Can you work these out from the model? Positions are in its coordinate system, mm. Round coordinates to 2 decimals unless told otherwise and drop trailing zeros. Loops run counter-clockwise (first coordinate to the right, second up) from the corner with the lowest first, then second, coordinate; pieces in that order, holes last.
from build123d import *

# Parameters (mm, degrees)
F0_R     = 1.2446
F0_R_2   = 1.2192
F0_R_3   = 4.445
F1_DEPTH = 1.016


with BuildPart() as f1:
    # F0 (on Top) → F1 (new body)
    with BuildSketch(Plane.XY):
        with BuildLine():
            ThreePointArc((13.305479, -78.509091), (15.141437, -76.814431), (17.563232, -76.2))
            Line((17.563232, -76.2), (17.145, -76.2))
            ThreePointArc((17.145, -76.2), (20.737102, -74.712102), (22.225, -71.12))
            Line((22.225, -71.12), (22.225, 71.12))
            ThreePointArc((22.225, 71.12), (20.737102, 74.712102), (17.145, 76.2))
            Line((17.145, 76.2), (17.563232, 76.2))
            ThreePointArc((17.563232, 76.2), (15.141437, 76.814431), (13.305479, 78.509091))
            ThreePointArc((13.305479, 78.509091), (0, 85.725), (-13.305479, 78.509091))
            ThreePointArc((-13.305479, 78.509091), (-15.141437, 76.814431), (-17.563232, 76.2))
            Line((-17.563232, 76.2), (-17.145, 76.2))
            ThreePointArc((-17.145, 76.2), (-20.737102, 74.712102), (-22.225, 71.12))
            Line((-22.225, 71.12), (-22.225, -71.12))
            ThreePointArc((-22.225, -71.12), (-20.737102, -74.712102), (-17.145, -76.2))
            Line((-17.145, -76.2), (-17.563232, -76.2))
            ThreePointArc((-17.563232, -76.2), (-15.141437, -76.814431), (-13.305479, -78.509091))
            ThreePointArc((-13.305479, -78.509091), (0, -85.725), (13.305479, -78.509091))
        make_face()
        with Locations((-11.43, -69.85)):
            Circle(F0_R, mode=Mode.SUBTRACT)
        with Locations((-15.875, -57.15)):
            Circle(F0_R_2, mode=Mode.SUBTRACT)
        with Locations((-15.875, -20.32)):
            Circle(F0_R_2, mode=Mode.SUBTRACT)
        with Locations((0, -80.645)):
            Circle(F0_R_2, mode=Mode.SUBTRACT)
        with Locations((0, -69.85)):
            Circle(F0_R_3, mode=Mode.SUBTRACT)
        with Locations((11.43, -69.85)):
            Circle(F0_R, mode=Mode.SUBTRACT)
        with Locations((15.875, -57.15)):
            Circle(F0_R_2, mode=Mode.SUBTRACT)
        with Locations((15.875, -20.32)):
            Circle(F0_R_2, mode=Mode.SUBTRACT)
        with Locations((-15.875, 20.32)):
            Circle(F0_R_2, mode=Mode.SUBTRACT)
        with Locations((-15.875, 57.15)):
            Circle(F0_R_2, mode=Mode.SUBTRACT)
        with Locations((-11.43, 69.85)):
            Circle(F0_R, mode=Mode.SUBTRACT)
        with Locations((15.875, 20.32)):
            Circle(F0_R_2, mode=Mode.SUBTRACT)
        with Locations((0, 69.85)):
            Circle(F0_R_3, mode=Mode.SUBTRACT)
        with Locations((0, 80.645)):
            Circle(F0_R_2, mode=Mode.SUBTRACT)
        with Locations((15.875, 57.15)):
            Circle(F0_R_2, mode=Mode.SUBTRACT)
        with Locations((11.43, 69.85)):
            Circle(F0_R, mode=Mode.SUBTRACT)
    extrude(amount=F1_DEPTH)


solid = f1.part
(1) If I drill on line 1 (Y direction, x = 0, z = 0.65) (3 decimals); line 2 (Y direction, x = -15.5, z = 0.6); line 3 (X direction, y = -69, z = 0.5) (3 decimals), over which ranges is the centre line in solid material (lowest first)?
Worked answers:
line 1: y = -85.725 to -81.864, -79.426 to -74.295, -65.405 to 65.405, 74.295 to 79.426, 81.864 to 85.725
line 2: y = -76.64 to -58.31, -55.99 to -21.48, -19.16 to 19.16, 21.48 to 55.99, 58.31 to 76.64
line 3: x = -22.225 to -12.339, -10.521 to -4.363, 4.363 to 10.521, 12.339 to 22.225
(2) If we section it at B-B, the plane x = 8: List the corners of the cut face in (y, z) for me.
Worked answers:
outline: (-83.56, 0) - (83.56, 0) - (83.56, 1.02) - (-83.56, 1.02) - close
(3) If we section it at A-A, the plane z = 0.55: State how many separate pieces and enclosed holes the cut face has, then the cut area to 3 significant figures.
Worked answers:
separate pieces: 1
enclosed holes: 16
area: 6,970 mm2
(4) If we mould it in two halves opening along Y, with no side actions, what happens to faces 1 (the cylindrical face through (0.221, 85.723, 0.501)), 2 (the cylindrical face through (-0.579, -65.443, 0.501)), 3 (the cylindrical face through (-0.221, -85.723, 0.501))? For each: released by +Y, released by -Y, zero draft, split by the parting line, or undercut.
Worked answers:
face 1: released by +Y
face 2: undercut
face 3: released by -Y
